Work out the finished part from the listing and answer in its coordinate system (mm). A direction names the side the tool comes from. Round coordinates to 2 decimals unless told otherwise and drop trailing zeros. Write each loop counter-clockwise with the first axis right and the second up, starting at its lowest first coordinate (ties: lowest second). Pieces come first, ordered by that corner, then holes. Notation, with made-up numbers: (18.25, -22) -> (73.25, -22) arc R19 ccw to (73.25, -13) -> close; hole circle Ø11 at (-26.75, 74.5). An arc over 180 degrees is marked (long way). One line per item, written item: value.
```python
from build123d import *

# Parameters (mm, degrees)
F0_R     = 12.7
F1_DEPTH = 63.5
F2_DEPTH = 76.2
F3_W     = 25.4
F3_H     = 25.4
F4_DEPTH = 12.7


with BuildPart() as f1:
    # F0 (on Front) → F1 (new body)
    with BuildSketch(Plane.XZ):
        Polygon((-12.7, 44.45), (-76.2, 44.45), (-76.2, -44.45), (76.2, -44.45), (76.2, 44.45), (12.7, 44.45), align=None)
        Circle(F0_R, mode=Mode.SUBTRACT)
    extrude(amount=F1_DEPTH)

    # F0 (on Front) → F2 (join)
    with BuildSketch(Plane.XZ):
        Circle(F0_R)
    extrude(amount=F2_DEPTH)

    # F3 (on Right) → F4 (join, symmetric)
    with BuildSketch(Plane.YZ):
        Polygon((-44.45, 44.316916), (-63.5, 44.316916), (-63.5, -44.583084), (0, -44.583084), (0, 44.316916), (-19.05, 44.316916), align=None)
        with Locations((-31.75, 57.016916)):
            Rectangle(F3_W, F3_H)
    extrude(amount=F4_DEPTH, both=True)


solid = f1.part
```
(1) Find section D-D on x = -63.5. Give the vertices of the cut face in (y, z).
Reported:
outline: (-63.5, -44.45) -> (0, -44.45) -> (0, 44.45) -> (-63.5, 44.45) -> close
(2) Consider probe 1 along Y at (x, z) = (-29.5, -27); probe 2 along Z at (x, y) = (67.5, -62); probe 3 along Z at (x, y) = (6, -52). Determine where each line is inside the solid, lowest interval first.
Reported:
probe 1: y = -63.5 to 0
probe 2: z = -44.45 to 44.45
probe 3: z = -44.58 to 44.45
(3) A tool of negligible diameter and unlimited length cuts with its end or side. For faces 1 (the face through (-45, -31, -44.45)), 2 (the face through (12.7, -32, 57)), 3 (the face through (0, -19.05, 57)), 4 (the face through (0, -44.45, 57)), from which of +Z, -Z, +X, -X, +Y, -Y can it reach the whole face along a straight path? Write none if from no direction.
Reported:
face 1: -Z, -X, +Y, -Y
face 2: +Z, +X, +Y, -Y
face 3: +Z, +X, -X, +Y
face 4: +Z, +X, -X, -Y
(4) Flat-ended cylindrical pins translate along their axes: pin 1 Ø1.5 at (x, y) = (43.5, -19) entering from +Z; pin 2 Ø12.5 at (x, z) = (-5, 51) entering from -Y; pin 3 Ø20 at (y, z) = (-34, 61) entering from -X. Find the tip coordinate at first contact, or state that the pin passes through.
Reported:
pin 1: stops at z = 44.45
pin 2: stops at y = -44.45
pin 3: stops at x = -12.7
(5) Find section B-B on y = -55.5. Give the vertices of the cut face in (x, z).
Reported:
outline: (-76.2, -44.45) -> (-12.7, -44.45) -> (-12.7, -44.58) -> (12.7, -44.58) -> (12.7, -44.45) -> (76.2, -44.45) -> (76.2, 44.45) -> (-76.2, 44.45) -> close
(6) Find section C-C on x = 0. Give the vertices of the cut face in (y, z).
Reported:
outline: (-76.2, -12.7) -> (-63.5, -12.7) -> (-63.5, -44.58) -> (0, -44.58) -> (0, 44.45) -> (-19.05, 44.45) -> (-19.05, 69.72) -> (-44.45, 69.72) -> (-44.45, 44.45) -> (-63.5, 44.45) -> (-63.5, 12.7) -> (-76.2, 12.7) -> close
(7) Find section A-A on z = 0. Give the vertices of the cut face in (x, y), plus the area to 4 significant figures.
Reported:
outline: (-76.2, -63.5) -> (-12.7, -63.5) -> (-12.7, -76.2) -> (12.7, -76.2) -> (12.7, -63.5) -> (76.2, -63.5) -> (76.2, 0) -> (-76.2, 0) -> close
area: 10,000 mm2
